For this review, take the finished solid that the model builds, in its own axes (mm). Face numbers are marked on the shaded views. A direction names the side the tool comes from. Coordinates: 2 decimals unless noted, no trailing zeros. Order: outer loops, then holes, each group sorted by start corner. A loop starts at its lowest first (then second) coordinate and runs counter-clockwise, first axis right, second up. Notation, with made-up numbers: (-32.5, 60) - (14.5, 60) arc R31 ccw to (14.5, 88) - close; hole circle Ø3 at (52, 87.25). An arc over 180 degrees is marked (long way). One line per item, written item: value. Start each with the question number.
(1) Clearance check with flat-ended pins moving along their axes: pin 1 (20 mm diameter, centred on x = -43.5, z = -56.5, fed in from +Y); pin 2 (4 mm diameter, centred on y = 18.5, z = -104.5, fed in from +X); pin 3 (4 mm diameter, centred on y = 123, z = -111, fed in from +X). State where each tip first meets the part, or that it passes through.
(2) To check wall thickness, follow line 1 along Z through (x, y) = (-28.65, 123); line 2 along Z through (x, y) = (-3.75, 2.65); line 3 along X through (y, z) = (2.2, -3.75). State the ranges of each line that lie inside material, in increasing order.
(3) Consider section D-D on x = -18.5. Write out the cut boundary in (y, z), then the cut area to 3 significant figures.
(4) Consider section C-C on y = 56.5. Write out the cut boundary in (x, z).
(5) Consider section A-A on x = -37. Write out the cut boundary in (y, z).
(6) Consider section B-B on z = -128. Write out the cut boundary in (x, y).
(7) For the marked faces 1, 2 and 3, list the 3-axis set-ups (+Z, -Z, +X, -X, +Y, -Y) from which the entire face can be reached by the end or side of a thin tool; tool diameter is ignored.
(8) Mouldability with a two-part tool opening along Z and no side actions: class the marked faces 4, 5, 6 and 7 as released by +Z, released by -Z, zero draft, split by the parting line, or undercut.
Autodesk Inventor part; units mm, degrees
ref_plane "YZ Plane" through (0, 0, 0) normal (1, 0, 0) x (0, 1, 0)
ref_plane "XZ Plane" through (0, 0, 0) normal (0, 1, 0) x (-1, 0, 0)
ref_plane "XY Plane" through (0, 0, 0) normal (0, 0, 1) x (1, 0, 0)
sketch "Sketch1" plane through (0, 0, 0) normal (0, 1, 0) x (-1, 0, 0)
  line L0 (0, 0) -> (46, 0)
  line L1 (0, -135) -> (0, 0)
  line L2 (0, 0) -> (50, 0)
  line L3 (50, 0) -> (50, -140)
  line L4 (50, -140) -> (0, -140)
  line L5 (0, -140) -> (0, 0)
  dimension "d36" = 50
  dimension "d37" = 140
extrude "Extrusion1" add sketch "Sketch1" along normal blind 5
sketch "Sketch2" plane through (0, 5, 0) normal (0, 1, 0) x (1, 0, 0)
  line L0 (0, 2.5) -> (17, 2.5) construction
  circle A0 centre (-3.75, 136.25) radius 1.5
  circle A1 centre (-46.25, 136.25) radius 1.5
  line L1 (0, 0) -> (-3.75, 0)
  circle A2 centre (-3.75, 3.75) radius 1.5
  circle A3 centre (-46.25, 3.75) radius 1.5
  point P0 (0, 135)
  point P1 (-50, 140)
  point P2 (0, 140)
  dimension "d103" = 3
  dimension "d106" = 3
  dimension "d109" = 3
  dimension "d110" = 3
extrude "Extrusion4" cut sketch "Sketch2" against normal through all
sketch "Sketch3" plane through (0, 5, 0) normal (0, 1, 0) x (1, 0, 0)
  line L0 (0, 0) -> (0, 140)
  line L1 (0, 70) -> (-25, 70)
  line L2 (0, 140) -> (-50, 140)
  line L3 (-25, 70) -> (-30, 70)
  line L4 (-30, 115) -> (-30, 70)
  line L5 (-30, 25) -> (-30, 70)
  line L6 (-30, 115) -> (-25, 115)
  line L7 (-25, 115) -> (-25, 25)
  line L8 (-25, 25) -> (-30, 25)
  line L9 (-30, 25) -> (-30, 115)
  line L10 (-25, 115) -> (-30, 115)
  line L11 (-30, 115) -> (-30, 120)
  line L12 (-30, 120) -> (-25, 120)
  line L13 (-25, 120) -> (-25, 115)
  line L14 (-25, 25) -> (-30, 25)
  line L15 (-30, 25) -> (-30, 20)
  line L16 (-30, 20) -> (-25, 20)
  line L17 (-25, 20) -> (-25, 25)
  dimension "d55" = 5
  dimension "d56" = 5
extrude "Extrusion5" add sketch "Sketch3" along normal blind 130
sketch "Sketch5" plane through (-30, 5, -120) normal (-1, 0, 0) x (0, 0, 1)
  line L0 (100, 0) -> (100, 130)
  line L1 (120, 0) -> (-20, 0)
  circle A0 centre (9.0002, 118) radius 1.5
  circle A1 centre (91.0002, 118) radius 1.5
  circle A2 centre (91.0002, 10) radius 1.5
  circle A3 centre (9.0002, 10) radius 1.5
  point P0 (120, -5)
  dimension "d62" = 3
  dimension "d63" = 3
  dimension "d64" = 3
  dimension "d65" = 3
extrude "Extrusion6" cut sketch "Sketch5" against normal up to surface (5 mm away)
sketch "Sketch6" plane through (-30, 5, -120) normal (-1, 0, 0) x (0, 0, 1)
  line L0 (0, 0) -> (3, 0)
  line L1 (3, 0) -> (3, 40)
  line L2 (3, 40) -> (0, 40)
  line L3 (0, 40) -> (0, 0)
  line L4 (100, 0) -> (0, 0)
  line L5 (100, 0) -> (97, 0)
  line L6 (97, 0) -> (97, 40)
  line L7 (97, 40) -> (100, 40)
  line L8 (100, 40) -> (100, 0)
  point P0 (120, -5)
  dimension "d68" = 3
  dimension "d69" = 40
  dimension "d70" = 3
  dimension "d71" = 40
extrude "Extrusion7" add sketch "Sketch6" along normal blind 20 and the other way blind 30
sketch "Sketch7" plane through (0, 5, -120) normal (0, 0, -1) x (-1, 0, 0)
  line L0 (0, 40) -> (25, 40)
  line L1 (50, 0) -> (50, 40)
  line L2 (0, 40) -> (50, 40)
  line L3 (50, 40) -> (50, 0)
  line L4 (50, 0) -> (0, 0)
  line L5 (0, 0) -> (0, 40)
  line L6 (50, 0) -> (0, 0)
  line L7 (25, 40) -> (0, 0)
  line L8 (30, 40) -> (50, 0)
  point P0 (0, -5)
sketch "Sketch8" plane through (-50, 5, -20) normal (0, 0, 1) x (1, 0, 0)
  line L0 (20, 40) -> (0, 40)
  line L1 (50, 40) -> (50, 0)
  line L2 (0, 40) -> (50, 40)
  line L3 (50, 40) -> (50, 0)
  line L4 (50, 0) -> (0, 0)
  line L5 (0, 0) -> (0, 40)
  line L6 (20, 40) -> (0, 0)
  line L7 (50, 40) -> (25, 40)
  line L8 (25, 40) -> (50, 0)
  point P0 (50, -5)
extrude "Extrusion8" cut sketch "Sketch8" against normal up to surface (3 mm away) contours L6 L5 L0 | L2 L1 L8
extrude "Extrusion9" cut sketch "Sketch7" against normal up to surface (3 mm away) contours L0 L7 L5 | L2 L1 L8
fillet "Fillet1" radius 2 8 edges at (-30, 5, -70) (-25, 5, -70) (-12.5, 5, -117) (-40, 5, -117) (-40, 5, -23) (-12.5, 5, -23) (-25, 5, -20) (-25, 5, -120)
thread "Thread5"
thread "Thread6"
thread "Thread7"
thread "Thread8"
fillet "Fillet2" radius 2 8 edges at (-30.5858, 5.5858, -23.5858) (-30, 26, -23) (-30.5858, 5.5858, -116.4142) (-30, 26, -117) (-24.4142, 5.5858, -116.4142) (-25, 26, -117) (-24.4142, 5.5858, -23.5858) (-25, 26, -23)
chamfer "Chamfer1" distance 1.5 angle 45 8 edges at (-25, 123, -30.4998) (-25, 123, -112.4998) (-25, 15, -112.4998) (-25, 15, -30.4998) (-5.25, 5, -136.25) (-47.75, 5, -136.25) (-5.25, 5, -3.75) (-47.75, 5, -3.75)
chamfer_without_effect "Chamfer2"
thread "Thread13"
thread "Thread14"
thread "Thread15"
thread "Thread16"
properties part number "support"
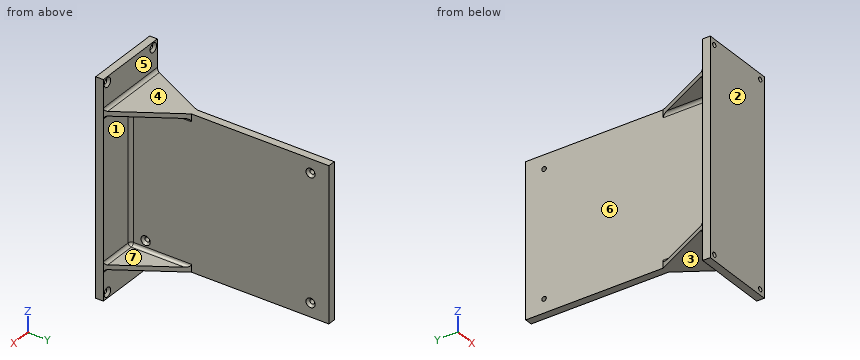
Geometry check:
1. pin 1: stops at y = 5
1. pin 2: stops at x = -25
1. pin 3: stops at x = -26
2. line 1: z = -120 to -112.5, -109.5 to -30.5, -27.5 to -20
2. line 2: z = -140 to -137.75, -134.75 to -5.25, -2.25 to 0
2. line 3: x = -50 to -47.75, -44.75 to -5.25, -2.25 to 0
3. outline: (0, -140) - (5, -140) - (5, -122) arc R2 cw to (7, -120) - (34.6, -120) - (34.6, -117) - (7, -117) arc R2 cw to (5, -115) - (5, -25) arc R2 cw to (7, -23) - (34.6, -23) - (34.6, -20) - (7, -20) arc R2 cw to (5, -18) - (5, 0) - (0, 0) - close
3. area: 881 mm^2
4. outline: (-30, -120) - (-25, -120) - (-25, -20) - (-30, -20) - close
5. outline: (0, -140) - (5, -140) - (5, -122) arc R2 cw to (7, -120) - (31, -120) - (31, -117) - (7, -117) arc R2 cw to (5, -115) - (5, -25) arc R2 cw to (7, -23) - (31, -23) - (31, -20) - (7, -20) arc R2 cw to (5, -18) - (5, 0) - (0, 0) - close
6. outline: (-50, 0) - (0, 0) - (0, 5) - (-50, 5) - close
7. face 1: +X, +Y
7. face 2: +Z, -Z, +X, -X, -Y
7. face 3: -Z, +X, -X, +Y
8. face 4: released by +Z
8. face 5: zero draft
8. face 6: undercut
8. face 7: undercut
